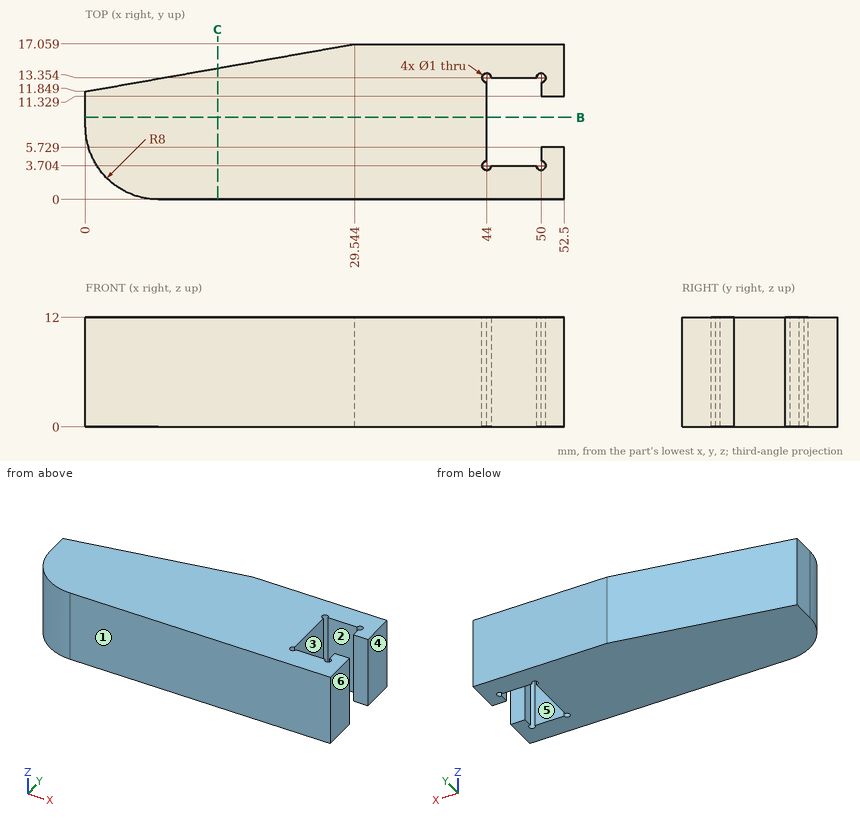
Design review of the part shown in the three views and the two pictorial views. Dimensions are in mm from the part's minimum x, y and z. A direction names the side the tool comes from. Round coordinates to 2 decimals unless told otherwise and drop trailing zeros. Write each loop counter-clockwise with the first axis right and the second up, starting at its lowest first coordinate (ties: lowest second). Pieces come first, ordered by that corner, then holes. Notation, with made-up numbers: (21, 45.25) -> (74, 45.25) arc R25 cw to (74, 81.25) -> close; hole circle Ø7 at (-16, -14). An arc over 180 degrees is marked (long way). One line per question, with ' | ' between items. Start each with the question number.
1) For pin 1 Ø1.2 at (y, z) = (5, 7) entering from -X, flat-tipped, find the tip position at first contact; note if it passes through.
2) Machinability: for the marked faces 5 and 6, which of the approach directions +Z, -Z, +X, -X, +Y, -Y give a long, thin tool a straight path to every point of the face, cutting with its end or side? Answer none if there is none.
3) Wall thickness on line 1 along Y through (x, z) = (47, 4.75) (1 decimal); line 2 along X through (y, z) = (3.75, 3.5); line 3 along X through (y, z) = (9, 1.25): over which ranges is each line inside the solid? List them lowest first.
4) Mouldability with a two-part tool opening along Y and no side actions: class the marked faces 1, 2, 3 and 4 as +Y half, -Y half, draft (parallel to the pull), parting line (faces both ways), or undercut.
5) Add section B-B (y = 9). Write out the cut boundary in (x, z), and give its area (3 significant figures).
6) Add section C-C (x = 14.5). Write out the cut boundary in (y, z).
Reported:
1) pin 1: stops at x = 0.37
2) face 5: +Z, -Z | face 6: +Z, -Z, +X, +Y, -Y
3) line 1: y = 0 to 3.7, 13.4 to 17.1 | line 2: x = 1.22 to 43.5, 50.5 to 52.5 | line 3: x = 0 to 44
4) face 1: -Y half | face 2: undercut | face 3: undercut | face 4: draft
5) outline: (0, 0) -> (44, 0) -> (44, 12) -> (0, 12) -> close | area: 528 mm²
6) outline: (0, 0) -> (14.41, 0) -> (14.41, 12) -> (0, 12) -> close
